```python
from build123d import *

# Parameters (mm, degrees)
PAD013_DEPTH = 5.7
PAD014_DEPTH = 2.5
PAD015_DEPTH = 0.5
PAD015_TAPER = 45


with BuildPart() as part:
    # Sketch028 (on Face271 of Binder002) → Pad013 (new body)
    with BuildSketch(Plane(origin=(0, 0, 0), x_dir=(0, -1, 0), z_dir=(-1, 0, 0))):
        with BuildLine():
            Line((-44.85, 89.1), (-44.85, 84.6))
            ThreePointArc((-44.85, 84.6), (-44.63033, 84.06967), (-44.1, 83.85))
            Line((-44.1, 83.85), (-39.6, 83.85))
            ThreePointArc((-39.6, 83.85), (-39.06967, 84.06967), (-38.85, 84.6))
            Line((-38.85, 84.6), (-38.85, 89.1))
            ThreePointArc((-38.85, 89.1), (-39.06967, 89.63033), (-39.6, 89.85))
            Line((-39.6, 89.85), (-44.1, 89.85))
            ThreePointArc((-44.1, 89.85), (-44.63033, 89.63033), (-44.85, 89.1))
        make_face()
    extrude(amount=-PAD013_DEPTH)

    # Sketch029 (on Face4 of Pad013) → Pad014 (join)
    with BuildSketch(Plane.YZ.offset(5.7)):
        with BuildLine():
            Line((38.85, 89.1), (38.85, 84.6))
            ThreePointArc((38.85, 84.6), (39.582233, 82.832233), (41.35, 82.1))
            Line((41.35, 82.1), (44.1, 82.1))
            ThreePointArc((44.1, 82.1), (45.867767, 82.832233), (46.6, 84.6))
            Line((46.6, 84.6), (46.6, 89.1))
            ThreePointArc((46.6, 89.1), (45.867767, 90.867767), (44.1, 91.6))
            Line((44.1, 91.6), (41.35, 91.6))
            ThreePointArc((41.35, 91.6), (39.582233, 90.867767), (38.85, 89.1))
        make_face()
    extrude(amount=PAD014_DEPTH)

    # Sketch028 (on Face271 of Binder002) → Pad015 (join)
    with BuildSketch(Plane(origin=(0, 0, 0), x_dir=(0, -1, 0), z_dir=(-1, 0, 0))):
        with BuildLine():
            Line((-44.85, 89.1), (-44.85, 84.6))
            ThreePointArc((-44.85, 84.6), (-44.63033, 84.06967), (-44.1, 83.85))
            Line((-44.1, 83.85), (-39.6, 83.85))
            ThreePointArc((-39.6, 83.85), (-39.06967, 84.06967), (-38.85, 84.6))
            Line((-38.85, 84.6), (-38.85, 89.1))
            ThreePointArc((-38.85, 89.1), (-39.06967, 89.63033), (-39.6, 89.85))
            Line((-39.6, 89.85), (-44.1, 89.85))
            ThreePointArc((-44.1, 89.85), (-44.63033, 89.63033), (-44.85, 89.1))
        make_face()
    extrude(amount=PAD015_DEPTH, taper=PAD015_TAPER)


solid = part.part
```
Model file for the job. Use its own axes, mm. A direction names the side the tool comes from. Give positions to 0.01 mm unless a question says otherwise; leave off trailing zeros. Loops run counter-clockwise (first coordinate to the right, second up) from the corner with the lowest first, then second, coordinate; pieces in that order, holes last. Notation, with made-up numbers: (-13, -24) -> (26, -24) arc R31 ccw to (26, 10) -> close; hole circle Ø1 at (63, 42.5). An arc over 180 degrees is marked (long way). Write each question's results on one line, items separated by ' | '.
(1) Tool access for faces 1 (the flat face through (8.2, 43, 87)), 2 (the cylindrical face through (6.932, 39.602, 90.887)), 3 (the flat face through (3, 44.85, 87)), 4 (the flat face through (3, 42, 89.85)), 5 (the flat face through (3, 42, 83.85)): list every direction of +Z, -Z, +X, -X, +Y, -Y with a clear straight run to the whole face (end or side of a thin tool).
Geometry results:
face 1: +Z, -Z, +X, +Y, -Y | face 2: +Z, +X, -X, -Y | face 3: +Z, -Z, -X, +Y | face 4: +Z, -X, +Y, -Y | face 5: -Z, -X, +Y, -Y
(2) Cut at D-D on y = 46.25. List the corners of the cut face in (x, z), and give its area (3 significant figures).
Geometry results:
outline: (5.7, 83.32) -> (8.2, 83.32) -> (8.2, 90.38) -> (5.7, 90.38) -> close | area: 17.6 mm²
(3) Cut at B-B on x = 6.5. List the corners of the cut face in (y, z).
Geometry results:
outline: (38.85, 84.6) arc R2.5 ccw to (41.35, 82.1) -> (44.1, 82.1) arc R2.5 ccw to (46.6, 84.6) -> (46.6, 89.1) arc R2.5 ccw to (44.1, 91.6) -> (41.35, 91.6) arc R2.5 ccw to (38.85, 89.1) -> close
(4) Cut at A-A on x = 1.25. List the corners of the cut face in (y, z).
Geometry results:
outline: (38.85, 84.6) arc R0.75 ccw to (39.6, 83.85) -> (44.1, 83.85) arc R0.75 ccw to (44.85, 84.6) -> (44.85, 89.1) arc R0.75 ccw to (44.1, 89.85) -> (39.6, 89.85) arc R0.75 ccw to (38.85, 89.1) -> close
(5) Probe line 1 along X through (y, z) = (46.25, 89.5); line 2 along Z through (x, y) = (0.25, 42.75); line 3 along Y through (x, z) = (7.5, 84.5). List the from-to ranges inside material, lowest first.
Geometry results:
line 1: x = 5.7 to 8.2 | line 2: z = 83.85 to 89.85 | line 3: y = 38.85 to 46.6
(6) Flat gauge pins, fed straight in: pin 1 Ø2 at (x, y) = (6.5, 45.5) entering from +Z; pin 2 Ø5 at (x, z) = (2, 86) entering from +Y; pin 3 Ø2 at (x, y) = (1.5, 41) entering from -Z. Where does each tip first touch, or does it go through?
Geometry results:
pin 1: stops at z = 91.57 | pin 2: stops at y = 44.85 | pin 3: stops at z = 83.85
(7) Cut at C-C on z = 90. List the corners of the cut face in (x, y).
Geometry results:
outline: (5.7, 39.02) -> (8.2, 39.02) -> (8.2, 46.43) -> (5.7, 46.43) -> close
